```python
from build123d import *

# Parameters (mm, degrees)
EXTRUDE_1_DEPTH     = 10
SKETCH_2_R          = 1.25
CUT_EXTRUDE_2_DEPTH = 13


with BuildPart() as part:
    # 草图1 → 凸台-拉伸1 (new body)
    with BuildSketch(Plane(origin=(0, 0, 0), x_dir=(1, 0, 0), z_dir=(0, 1, 0))):
        with BuildLine():
            Line((8, 0), (13, 0))
            Line((13, 0), (13, 10.5))
            Line((13, 10.5), (-13, 10.5))
            Line((-13, 10.5), (-13, 0))
            Line((-13, 0), (-8, 0))
            ThreePointArc((-8, 0), (0, 8), (8, 0))
        make_face()
    extrude(amount=EXTRUDE_1_DEPTH)

    # 草图2 → 切除-拉伸2 (cut)
    with BuildSketch(Plane(origin=(0, 0, -10.5), x_dir=(-1, 0, 0), z_dir=(0, 0, -1))):
        with Locations((-11, 5)):
            Circle(SKETCH_2_R)
        with Locations((0, 5)):
            Circle(SKETCH_2_R)
        with Locations((11, 5)):
            Circle(SKETCH_2_R)
    extrude(amount=-CUT_EXTRUDE_2_DEPTH, mode=Mode.SUBTRACT)


solid = part.part
```
Build history of the part. All positions in model axes, mm. Round coordinates to 2 decimals unless told otherwise and drop trailing zeros. Write each loop counter-clockwise with the first axis right and the second up, starting at its lowest first coordinate (ties: lowest second). Pieces come first, ordered by that corner, then holes.
1) Band-saw the part on C-C, the plane z = -4.25. List the corners of the cut face in (x, y).
2) Pin check, flat tips, straight feed: pin 1 (3 mm diameter, centred on x = 0, y = 5, fed in from +Z); pin 2 (1 mm diameter, centred on x = -2.5, z = -7, fed in from +Y); pin 3 (4 mm diameter, centred on x = -5, y = 4, fed in from +Z). Stop position of each tip, or through.
3) Band-saw the part on B-B, the plane y = 5. List the corners of the cut face in (x, z), and give its area (3 significant figures).
4) Drill centre lines: probe 1 along Y at (x, z) = (-11, -3.75); probe 2 along X at (y, z) = (4.25, -0.25); probe 3 along Z at (x, y) = (1.25, 1). Where is each one in solid material? Low to high.
5) Mould opens along Y. For faces 1 (the flat face through (0, 7, -10.5)), 2 (the cylindrical face through (-10.01, 4.24, -5.32)), 3 (the cylindrical face through (11.99, 4.24, -5.32)), 4 (the flat face through (0, 10, -9)) say: +Y half, -Y half, draft (parallel to the pull), parting line (faces both ways), or undercut.
6) Band-saw the part on A-A, the plane x = -11. List the corners of the cut face in (y, z).
7) Band-saw the part on D-D, the plane x = 0. List the corners of the cut face in (y, z), and give its area (4 significant figures).
Ans:
1. outline: (-13, 0) - (-6.78, 0) - (-6.78, 10) - (-13, 10) - close; (6.78, 0) - (13, 0) - (13, 10) - (6.78, 10) - close; hole circle Ø2.5 at (-11, 5); hole circle Ø2.5 at (11, 5)
2. pin 1: stops at z = -7.86
2. pin 2: passes through
2. pin 3: stops at z = -3.87
3. outline: (-13, -10.5) - (-12.25, -10.5) - (-12.25, 0) - (-13, 0) - close; (-9.75, -10.5) - (-1.25, -10.5) - (-1.25, -7.9) arc R8 cw to (-8, 0) - (-9.75, 0) - close; (1.25, -10.5) - (9.75, -10.5) - (9.75, 0) - (8, 0) arc R8 cw to (1.25, -7.9) - close; (12.25, -10.5) - (13, -10.5) - (13, 0) - (12.25, 0) - close
3. area: 114 mm2
4. probe 1: y = 0 to 3.75, 6.25 to 10
4. probe 2: x = -13 to -12, -10 to -8, 8 to 10, 12 to 13
4. probe 3: z = -10.5 to -7.9
5. face 1: draft
5. face 2: undercut
5. face 3: undercut
5. face 4: +Y half
6. outline: (0, -10.5) - (3.75, -10.5) - (3.75, 0) - (0, 0) - close; (6.25, -10.5) - (10, -10.5) - (10, 0) - (6.25, 0) - close
7. outline: (0, -10.5) - (3.75, -10.5) - (3.75, -8) - (0, -8) - close; (6.25, -10.5) - (10, -10.5) - (10, -8) - (6.25, -8) - close
7. area: 18.75 mm2
